from build123d import *

# Parameters (mm, degrees)
BOSS_EXTRUDE1_DEPTH                                  = 50.8
SKETCH2_W                                            = 20
SKETCH2_H                                            = 55
CUT_EXTRUDE1_DEPTH                                   = 1485.951393144
SKETCH3_W                                            = 50.8
SKETCH3_H                                            = 5
CUT_EXTRUDE2_DEPTH                                   = 1553.894278436
SKETCH5_W                                            = 115
SKETCH5_H                                            = 323.205505282
CUT_EXTRUDE5_DEPTH                                   = 5
CUT_EXTRUDE6_START                                   = -27
SKETCH6_W                                            = 185
SKETCH6_H                                            = 150
CUT_EXTRUDE6_DEPTH                                   = 1458.401778495
FILLET1_R                                            = 38.1
M12_TAPPED_HOLE1_D                                   = 10.2
M12_TAPPED_HOLE1_DEPTH                               = 43.99
M12_TAPPED_HOLE1_TIP                                 = 3.064389157
CUT_EXTRUDE7_DEPTH                                   = 5.08
CBORE_FOR_M12_HEX_SOCKET_HEAD_CAP_SCREW1_D           = 13.5
CBORE_FOR_M12_HEX_SOCKET_HEAD_CAP_SCREW1_CBORE_D     = 20
CBORE_FOR_M12_HEX_SOCKET_HEAD_CAP_SCREW1_CBORE_DEPTH = 13
M12_TAPPED_HOLE2_D                                   = 10.2
M12_TAPPED_HOLE2_DEPTH                               = 43.99
M12_TAPPED_HOLE2_TIP                                 = 3.064389157
FILLET2_R                                            = 0.79375
FILLET3_R                                            = 0.79375
SKETCH16_W                                           = 225
SKETCH16_H                                           = 50.8
SKETCH16_W_2                                         = 50.8
SKETCH16_H_2                                         = 195.8
CUT_EXTRUDE8_DEPTH                                   = 1485.788752654
SKETCH17_R                                           = 31.75
SKETCH17_W                                           = 3.175
SKETCH17_H                                           = 38.1
CUT_EXTRUDE9_DEPTH                                   = 1485.951393147
SKETCH18_R                                           = 31.75
CUT_EXTRUDE10_DEPTH                                  = 1485.951393147


with BuildPart() as part:
    # Sketch1 → Boss-Extrude1 (new body)
    with BuildSketch(Plane(origin=(0, 0, 0), x_dir=(0, 0, -1), z_dir=(1, 0, 0))):
        with BuildLine():
            Line((0, 350), (0, 1129.289321881))
            ThreePointArc((0, 1129.289321881), (-3.806023374, 1148.4234935), (-14.644660941, 1164.644660941))
            Line((-14.644660941, 1164.644660941), (-85.355339059, 1235.355339059))
            ThreePointArc((-85.355339059, 1235.355339059), (-101.5765065, 1246.193976626), (-120.710678119, 1250))
            Line((-120.710678119, 1250), (-175, 1250))
            ThreePointArc((-175, 1250), (-210.355339059, 1235.355339059), (-225, 1200))
            Line((-225, 1200), (-225, 807.842712475))
            ThreePointArc((-225, 807.842712475), (-240.224093498, 731.306026002), (-283.578643763, 666.421356237))
            Line((-283.578643763, 666.421356237), (-770.710678119, 179.289321881))
            ThreePointArc((-770.710678119, 179.289321881), (-792.387953251, 146.846986999), (-800, 108.578643763))
            Line((-800, 108.578643763), (-800, 0))
            Line((-800, 0), (0, 0))
            Line((0, 0), (120, 0))
            Line((120, 0), (120, 250))
            ThreePointArc((120, 250), (105.355339059, 285.355339059), (70, 300))
            Line((70, 300), (50, 300))
            ThreePointArc((50, 300), (14.644660941, 314.644660941), (0, 350))
        make_face()
    extrude(amount=BOSS_EXTRUDE1_DEPTH)

    # Sketch2 → Cut-Extrude1 (cut, through all)
    with BuildSketch(Plane(origin=(0, 1250, 0), x_dir=(1, 0, 0), z_dir=(0, 1, 0))):
        with Locations((40.8, -22.5)):
            Rectangle(SKETCH2_W, SKETCH2_H)
    extrude(amount=-CUT_EXTRUDE1_DEPTH, mode=Mode.SUBTRACT)

    # Sketch3 → Cut-Extrude2 (cut, through all)
    with BuildSketch(Plane(origin=(0, 0, 800), x_dir=(-1, 0, 0), z_dir=(0, 0, -1))):
        with Locations((-25.4, 2.5)):
            Rectangle(SKETCH3_W, SKETCH3_H)
    extrude(amount=CUT_EXTRUDE2_DEPTH, mode=Mode.SUBTRACT)

    # Sketch5 → Cut-Extrude5 (cut)
    with BuildSketch(Plane(origin=(50.8, 0, 0), x_dir=(0, 0, -1), z_dir=(1, 0, 0))):
        with Locations((62.5, 166.602752641)):
            Rectangle(SKETCH5_W, SKETCH5_H)
    extrude(amount=-CUT_EXTRUDE5_DEPTH, mode=Mode.SUBTRACT)

    # Sketch6 → Cut-Extrude6 (cut, through all)
    with BuildSketch(Plane(origin=(30.8, 0, 0), x_dir=(0, 0, -1), z_dir=(1, 0, 0)).offset(CUT_EXTRUDE6_START)):
        with Locations((-92.5, 520)):
            Rectangle(SKETCH6_W, SKETCH6_H)
    extrude(amount=-CUT_EXTRUDE6_DEPTH, mode=Mode.SUBTRACT)

    # Fillet1
    fillet1_edges = [part.edges().sort_by_distance(p)[0] for p in [
        (1.9, 445, 185),
        (1.9, 595, 185),
    ]]
    fillet(fillet1_edges, radius=FILLET1_R)

    # M12 Tapped Hole1
    with Locations(Plane.ZY.offset(-3.8)):
        with Locations((150, 561), (18, 561), (18, 481), (150, 481)):
            Hole(M12_TAPPED_HOLE1_D / 2, depth=M12_TAPPED_HOLE1_DEPTH)
            with Locations((0, 0, -(M12_TAPPED_HOLE1_DEPTH + M12_TAPPED_HOLE1_TIP / 2))):  # 118° drill point
                Cone(0, M12_TAPPED_HOLE1_D / 2, M12_TAPPED_HOLE1_TIP, mode=Mode.SUBTRACT)

    # Sketch9 → Cut-Extrude7 (cut)
    with BuildSketch(Plane.ZY.offset(-3.8)):
        with BuildLine():
            Line((95, 544), (95, 498))
            ThreePointArc((95, 498), (89, 492), (83, 498))
            Line((83, 498), (83, 544))
            ThreePointArc((83, 544), (89, 550), (95, 544))
        make_face()
    extrude(amount=-CUT_EXTRUDE7_DEPTH, mode=Mode.SUBTRACT)

    # CBORE for M12 Hex Socket Head Cap Screw1 (through all)
    with Locations(Plane.ZY):
        with Locations((20, 33), (-80, 58), (-80, 133), (-80, 208), (20, 133), (20, 233), (20, 333), (20, 433), (20, 533), (20, 633), (20, 733), (20, 833), (20, 933), (20, 1033)):
            CounterBoreHole(CBORE_FOR_M12_HEX_SOCKET_HEAD_CAP_SCREW1_D / 2, CBORE_FOR_M12_HEX_SOCKET_HEAD_CAP_SCREW1_CBORE_D / 2, CBORE_FOR_M12_HEX_SOCKET_HEAD_CAP_SCREW1_CBORE_DEPTH)

    # M12 Tapped Hole2
    with Locations(Plane(origin=(0, 5, 0), x_dir=(-1, 0, 0), z_dir=(0, -1, 0))):
        with Locations((-25.8, 90), (-25.8, 30), (-25.8, -60), (-25.8, -140), (-25.8, -220), (-25.8, -380), (-25.8, -300), (-25.8, -460), (-25.8, -540), (-25.8, -620), (-25.8, -710), (-25.8, -770)):
            Hole(M12_TAPPED_HOLE2_D / 2, depth=M12_TAPPED_HOLE2_DEPTH)
            with Locations((0, 0, -(M12_TAPPED_HOLE2_DEPTH + M12_TAPPED_HOLE2_TIP / 2))):  # 118° drill point
                Cone(0, M12_TAPPED_HOLE2_D / 2, M12_TAPPED_HOLE2_TIP, mode=Mode.SUBTRACT)

    # Fillet2
    fillet2_edges = [part.edges().sort_by_distance(p)[0] for p in [
        (8.88, 550, 89),
        (8.88, 521, 95),
        (8.88, 492, 89),
        (8.88, 521, 83),
    ]]
    fillet(fillet2_edges, radius=FILLET2_R)

    # Fillet3
    fillet3_edges = [part.edges().sort_by_distance(p)[0] for p in [
        (30.8, 602.5, 50),
        (30.8, 166.602752641, -5),
    ]]
    fillet(fillet3_edges, radius=FILLET3_R)

    # Sketch16 → Cut-Extrude8 (cut, through all)
    with BuildSketch(Plane(origin=(45.8, 0, 0), x_dir=(0, 0, -1), z_dir=(1, 0, 0))):
        with Locations((-112.5, 1224.6)):
            Rectangle(SKETCH16_W, SKETCH16_H)
        with Locations((-774.6, 102.9)):
            Rectangle(SKETCH16_W_2, SKETCH16_H_2)
    extrude(amount=CUT_EXTRUDE8_DEPTH, mode=Mode.SUBTRACT)

    # Sketch17 → Cut-Extrude9 (cut, through all)
    with BuildSketch(Plane(origin=(50.8, 0, 0), x_dir=(0, 0, -1), z_dir=(1, 0, 0))):
        with Locations((-139.6896, 144.2936)):
            Circle(SKETCH17_R)
        with Locations((118.4125, 24.05)):
            Rectangle(SKETCH17_W, SKETCH17_H)
    extrude(amount=-CUT_EXTRUDE9_DEPTH, mode=Mode.SUBTRACT)

    # Sketch18 → Cut-Extrude10 (cut, through all)
    with BuildSketch(Plane(origin=(50.8, 0, 0), x_dir=(0, 0, -1), z_dir=(1, 0, 0))):
        with Locations((-639.6896, 144.2936)):
            Circle(SKETCH18_R)
        with Locations((-139.6896, 1155)):
            Circle(SKETCH18_R)
    extrude(amount=-CUT_EXTRUDE10_DEPTH, mode=Mode.SUBTRACT)


solid = part.part
Work out the finished part from the listing and answer in its coordinate system (mm). A direction names the side the tool comes from. Give positions to 0.01 mm unless a question says otherwise; leave off trailing zeros. Order: outer loops, then holes, each group sorted by start corner. A loop starts at its lowest first (then second) coordinate and runs counter-clockwise, first axis right, second up. Notation, with made-up numbers: (-26, 27.25) -> (30, 27.25) arc R21 cw to (30, 37.25) -> close; hole circle Ø7 at (5, 59.25). An arc over 180 degrees is marked (long way). Answer as a JSON object with one key per item and string values. Group by question number.
1. Section A-A on y = 1009.5 is taken. Determine the outline of the cut face in (x, z), plus the area to 3 significant figures.
2. The mould has two halves that part along Y. Classify faces 1 (the flat face through (23, 58, 800)), 2 (the cylindrical face through (25.76, 145.69, 671.41)), 3 (the cylindrical face through (22.58, 147.35, 792.18)): released by +Y, released by -Y, zero draft, split by the parting line, or undercut.
3. Flat-ended cylindrical pins translate along their axes: pin 1 Ø16 at (y, z) = (233, 20) entering from -X; pin 2 Ø2 at (x, y) = (39.5, 1074.5) entering from +Z; pin 3 Ø1.5 at (x, y) = (34, 335.5) entering from +Z; pin 4 Ø12 at (y, z) = (208, -80) entering from -X. Find the tip coordinate at first contact, or state that the pin passes through.
4. Section B-B on y = 271 is taken. Determine the outline of the cut face in (x, z), plus the area to 3 significant figures.
5. Section C-C on z = 242 is taken. Determine the outline of the cut face in (x, y).
6. A tool of negligible diameter and unlimited length cuts with its end or side. For faces 4 (the flat face through (23, 24, -116.825)), 5 (the flat face through (15, 734, 0)), 6 (the cylindrical face through (1.87, 455.86, 173.54)), 7 (the flat face through (45.8, 1219, 139)), from which of +Z, -Z, +X, -X, +Y, -Y can it reach the whole face along a straight path? Write none if from no direction.
7. Consider line 1 along Y through (x, z) = (13.5, 144.5); line 2 along Z through (x, y) = (25.5, 933); line 3 along Z through (x, y) = (32.5, 905). Determine where each line is inside the solid, lowest interval first. Write a range as [from, to].
Result sheet:
{
 "1": {"outline": "(0, 0) -> (30.8, 0) -> (30.8, 49.21) arc R0.79 cw to (31.59, 50) -> (50.8, 50) -> (50.8, 225) -> (0, 225) -> close", "area": "10,400 mm^2"},
 "2": {"face 1": "zero draft", "face 2": "undercut", "face 3": "released by +Y"},
 "3": {"pin 1": "stops at x = 13", "pin 2": "stops at z = 225", "pin 3": "stops at z = 615.25", "pin 4": "passes through"},
 "4": {"outline": "(0, -115.38) -> (45.8, -115.38) -> (45.8, -5) -> (31.59, -5) arc R0.79 cw to (30.8, -4.21) -> (30.8, 49.21) arc R0.79 cw to (31.59, 50) -> (50.8, 50) -> (50.8, 679) -> (0, 679) -> close", "area": "38,700 mm^2"},
 "5": {"outline": "(0, 5) -> (50.8, 5) -> (50.8, 727.15) -> (0, 727.15) -> close"},
 "6": {"face 4": "-Z, +X, -X, -Y", "face 5": "-Z, +X, -X, +Y", "face 6": "-Z, -X", "face 7": "+Z, -Z, +X, +Y"},
 "7": {"line 1": "y = [5, 112.91], [175.68, 1123.62], [1186.38, 1250]", "line 2": "z = [0, 13.25], [26.75, 225]", "line 3": "z = [50, 225]"}
}
